from build123d import *

# Parameters (mm, degrees)
EXTRUDE_1_DEPTH     = 120
CUT_EXTRUDE_1_DEPTH = 2


with BuildPart() as part:
    # 草图2 → 凸台-拉伸1 (new body)
    with BuildSketch(Plane.XY):
        Polygon((0, 2), (16.856230065, 11.032475858), (19.332704549, 11.032475858), (2.476474484, 2), (10, 2), (26.856230065, 11.032475858), (29.332704549, 11.032475858), (12.476474484, 2), (20, 2), (36.856230065, 11.032475858), (39.332704549, 11.032475858), (22.476474484, 2), (30, 2), (46.856230065, 11.032475858), (49.332704549, 11.032475858), (32.476474484, 2), (40, 2), (56.856230065, 11.032475858), (59.332704549, 11.032475858), (42.476474484, 2), (50, 2), (66.856230065, 11.032475858), (69.332704549, 11.032475858), (52.476474484, 2), (60, 2), (76.856230065, 11.032475858), (79.332704549, 11.032475858), (62.476474484, 2), (70, 2), (86.856230065, 11.032475858), (89.332704549, 11.032475858), (72.476474484, 2), (80, 2), (96.856230065, 11.032475858), (99.332704549, 11.032475858), (82.476474484, 2), (90, 2), (106.856230065, 11.032475858), (109.332704549, 11.032475858), (92.476474484, 2), (100, 2), (116.856230065, 11.032475858), (119.332704549, 11.032475858), (102.476474484, 2), (110, 2), (126.856230065, 11.032475858), (129.332704549, 11.032475858), (112.476474484, 2), (120, 2), (120, 0), (0, 0), align=None)
    extrude(amount=EXTRUDE_1_DEPTH)

    # 草图5 → 切除-拉伸1 (cut)
    with BuildSketch(Plane.XZ):
        Polygon((2.476402921, 117.653523678), (2.48, 2.48), (10, 2.48), (9.999928921, 117.653523678), align=None)
        Polygon((19.996402921, 117.653523678), (12.472876921, 117.653523678), (12.476474, 2.48), (19.774552048, 2.48), (19.996474, 2.48), align=None)
        Polygon((32.465824921, 117.653523678), (32.469422, 2.48), (39.323656144, 2.48), (39.989422, 2.48), (39.989350921, 117.653523678), align=None)
        Polygon((42.462298921, 117.653523678), (42.465896, 2.48), (49.098208192, 2.48), (49.985896, 2.48), (49.985824921, 117.653523678), align=None)
        Polygon((52.458772921, 117.653523678), (52.46237, 2.48), (58.87276024, 2.48), (59.98237, 2.48), (59.982298921, 117.653523678), align=None)
        Polygon((62.455246921, 117.653523678), (62.458844, 2.48), (68.647312287, 2.48), (69.978844, 2.48), (69.978772921, 117.653523678), align=None)
        Polygon((72.451720921, 117.653523678), (72.455318, 2.48), (78.421864335, 2.48), (79.975318, 2.48), (79.975246921, 117.653523678), align=None)
        Polygon((82.448194921, 117.653523678), (82.451792, 2.48), (88.196416383, 2.48), (89.971792, 2.48), (89.971720921, 117.653523678), align=None)
        Polygon((92.444668921, 117.653523678), (92.448266, 2.48), (97.970968431, 2.48), (99.968266, 2.48), (99.968194921, 117.653523678), align=None)
        Polygon((102.441142921, 117.653523678), (102.44474, 2.48), (107.745520479, 2.48), (109.96474, 2.48), (109.964668921, 117.653523678), align=None)
        Polygon((22.469350921, 117.653523678), (22.472948, 2.48), (29.992948, 2.48), (29.992876921, 117.653523678), align=None)
    extrude(amount=-CUT_EXTRUDE_1_DEPTH, mode=Mode.SUBTRACT)


solid = part.part
For this review, take the finished solid that the model builds, in its own axes (mm). A direction names the side the tool comes from. Give positions to 0.01 mm unless a question says otherwise; leave off trailing zeros. Loops run counter-clockwise (first coordinate to the right, second up) from the corner with the lowest first, then second, coordinate; pieces in that order, holes last.
Item 1: Take a section at B-B, the plane z = 82.5. Give the number of separate pieces and of enclosed holes in the cut face, and give its area (3 significant figures).
Item 2: Take a section at A-A, the plane x = 15. State the section outline as (y, z) points.
Item 3: For line 1 along Z through (x, y) = (8, 1); line 2 along Y through (x, z) = (64, 55); line 3 along Y through (x, z) = (17.5, 93), list the stretches that pass through material, from the lowest coordinate up.
Item 4: Tool access review of faces 1 (the flat face through (65.6, 4.4, 0)), 2 (the flat face through (68.31, 6.453, 59.16)): name each direction out of +Z, -Z, +X, -X, +Y, -Y from which nothing blocks a thin tool from reaching the whole face with its end or side.
Item 5: Insertion check: pin 1 (8 mm diameter, centred on x = 113, z = 29.5, fed in from +Y); pin 2 (1 mm diameter, centred on y = 0.5, z = 63.5, fed in from +X); pin 3 (1 mm diameter, centred on y = 6, z = 41.5, fed in from -X). Each pin has a flat end and moves straight along its axis. Give the tip position at first contact, or say it passes through.
Item 6: Draft analysis for pull direction Y (two halves, no side actions). For faces 3 (the flat face through (61, 0, 59)), 4 (the flat face through (38.31, 6.453, 59.16)), 5 (the flat face through (65.6, 4.4, 120)), state which applies: +Y half, -Y half, draft (parallel to the pull), parting line (faces both ways), or undercut.
Calculated:
1. separate pieces: 12
1. enclosed holes: 0
1. area: 343 mm2
2. outline: (0, 0) - (2, 0) - (2, 2.48) - (0, 2.48) - close; (0, 117.65) - (2, 117.65) - (2, 120) - (0, 120) - close; (3.35, 0) - (4.68, 0) - (4.68, 120) - (3.35, 120) - close; (8.71, 0) - (10.04, 0) - (10.04, 120) - (8.71, 120) - close
3. line 1: z = 0 to 2.48, 117.65 to 120
3. line 2: y = 2.82 to 4.14, 8.17 to 9.5
3. line 3: y = 4.69 to 6.02, 10.05 to 11.03
4. face 1: -Z, +X, -X, +Y, -Y
4. face 2: +Z, -Z
5. pin 1: stops at y = 11.03
5. pin 2: stops at x = 120
5. pin 3: stops at x = 6.53
6. face 3: -Y half
6. face 4: undercut
6. face 5: draft
